Geometry check sheet. Reference: the model listing, model coordinates, mm. A direction names the side the tool comes from. Give positions to 0.01 mm unless a question says otherwise; leave off trailing zeros. Order: outer loops, then holes, each group sorted by start corner. A loop starts at its lowest first (then second) coordinate and runs counter-clockwise, first axis right, second up.
```python
from build123d import *

# Parameters (mm, degrees)
F0_W     = 45.5
F0_H     = 23
F0_W_2   = 41.5
F0_H_2   = 19
F1_DEPTH = 25
F0_W_3   = 61.5
F0_H_3   = 39
F2_DEPTH = 3
F3_R     = 2
F4_DEPTH = 3.001


with BuildPart() as f1:
    # F0 (on Top) → F1 (new body)
    with BuildSketch(Plane.XY):
        with Locations((-20.75, 9.5)):
            Rectangle(F0_W, F0_H)
        with Locations((-20.75, 9.5)):
            Rectangle(F0_W_2, F0_H_2, mode=Mode.SUBTRACT)
    extrude(amount=F1_DEPTH)

    # F0 (on Top) → F2 (join)
    with BuildSketch(Plane.XY):
        with Locations((-20.75, 9.5)):
            Rectangle(F0_W_3, F0_H_3)
        with Locations((-20.75, 9.5)):
            Rectangle(F0_W, F0_H, mode=Mode.SUBTRACT)
    extrude(amount=F2_DEPTH)

    # F3 (on face) → F4 (cut, through all)
    with BuildSketch(Plane.XY.offset(3)):
        with Locations((-46.968646, 24.716979)):
            Circle(F3_R)
        with Locations((-20.668646, 24.716979)):
            Circle(F3_R)
        with Locations((5.631354, 24.716979)):
            Circle(F3_R)
        with Locations((-46.968646, 9.299078)):
            Circle(F3_R)
        with Locations((5.631354, 9.299078)):
            Circle(F3_R)
        with Locations((-46.968646, -6.118824)):
            Circle(F3_R)
        with Locations((-20.668646, -6.118824)):
            Circle(F3_R)
        with Locations((5.631354, -6.118824)):
            Circle(F3_R)
    extrude(amount=-F4_DEPTH, mode=Mode.SUBTRACT)


solid = f1.part
```
Q1. Cross-section at B-B, the plane z = 21.25. Record the boundary of the cut face in (x, y), and give its area (3 significant figures).
Q2. Cross-section at D-D, the plane y = 22. Record the boundary of the cut face in (x, z), and give its area (4 significant figures).
Q3. Release check for a two-part mould opening along Y. For faces 5 (the face through (-43.5, 9, 14)), 6 (the face through (-45.1, 24, 1.5)), 7 (the face through (-21, 21, 14)) record: pulls with the +Y half, pulls with the -Y half, needs draft (parallel to the pull), parting line crosses it, or undercut.
Q4. Access from +Z, -Z, +X, -X, +Y, -Y to the whole of each face (thin tool, end or side, straight path). Record for faces 1 (the face through (2, 9, 14)), 2 (the face through (-21, -2, 14)), 3 (the face through (-23, -1, 25)), 4 (the face through (-41.5, 9, 12)).
Q5. Thickness scan on L1, parallel to Y at x = -13, z = 12.5; L2, parallel to X at y = 14, z = 18.5; L3, parallel to Y at x = -34.5, z = 2.75. Record the ranges inside material, lowest first.
Q6. Cross-section at A-A, the plane x = -26. Record the boundary of the cut face in (y, z).
Q7. Gauge pin test, flat ends, axial feed: P1, Ø5.5, axis at y = 6, z = 6.5, coming from the +X side; P2, Ø5, axis at x = -28, z = 12.5, coming from the -Y side; P3, Ø3, axis at x = -20.67, y = 24.72, coming from the -Z side; P4, Ø4.5, axis at x = -46.97, y = 24.72, coming from the +Z side. Record the tip position at first contact, or that the pin passes through.
Q8. Cross-section at C-C, the plane y = 10. Record the boundary of the cut face in (x, z).
Answers follow:
1. outline: (-43.5, -2) - (2, -2) - (2, 21) - (-43.5, 21) - close; hole (-41.5, 0) - (0, 0) - (0, 19) - (-41.5, 19) - close
1. area: 258 mm2
2. outline: (-51.5, 0) - (10, 0) - (10, 3) - (-51.5, 3) - close
2. area: 184.5 mm2
3. face 5: needs draft
3. face 6: undercut
3. face 7: pulls with the +Y half
4. face 1: +Z, +X, +Y, -Y
4. face 2: +Z, +X, -X, -Y
4. face 3: +Z, +X, -X, +Y, -Y
4. face 4: +Z, -Z
5. L1: y = -2 to 0, 19 to 21
5. L2: x = -43.5 to -41.5, 0 to 2
5. L3: y = -10 to 0, 19 to 29
6. outline: (-10, 0) - (0, 0) - (0, 25) - (-2, 25) - (-2, 3) - (-10, 3) - close; (19, 0) - (29, 0) - (29, 3) - (21, 3) - (21, 25) - (19, 25) - close
7. P1: stops at x = 2
7. P2: stops at y = -2
7. P3: passes through
7. P4: stops at z = 3
8. outline: (-51.5, 0) - (-48.84, 0) - (-48.84, 3) - (-51.5, 3) - close; (-45.1, 0) - (-41.5, 0) - (-41.5, 25) - (-43.5, 25) - (-43.5, 3) - (-45.1, 3) - close; (0, 0) - (3.76, 0) - (3.76, 3) - (2, 3) - (2, 25) - (0, 25) - close; (7.5, 0) - (10, 0) - (10, 3) - (7.5, 3) - close
